```python
from build123d import *

# Parameters (mm, degrees)
F1_DEPTH = 40
F2_T     = -5
F4_D     = 80
F4_DEPTH = 60


with BuildPart() as f1:
    # F0 (on Top) → F1 (new body)
    with BuildSketch(Plane.XY):
        Polygon((-170, 270), (-170, 0), (-170, -270), (170, -270), (170, 270), align=None)
    extrude(amount=F1_DEPTH)

    # F2
    f2_openings = [f1.faces().sort_by_distance(p)[0] for p in [
        (0, 0, 40),
    ]]
    offset(amount=F2_T, openings=f2_openings)

    # F4
    with Locations(Plane.XY.offset(5)):
        with Locations((120, 220)):
            Hole(F4_D / 2, depth=F4_DEPTH)


solid = f1.part
```
Could you check a few things on this model? Use its own coordinates, in mm. A direction names the side the tool comes from. Round coordinates to 2 decimals unless told otherwise and drop trailing zeros. Order: outer loops, then holes, each group sorted by start corner. A loop starts at its lowest first (then second) coordinate and runs counter-clockwise, first axis right, second up. Notation, with made-up numbers: (12, -24.75) -> (25, -24.75) arc R25 ccw to (25, 14.25) -> close; hole circle Ø11 at (79, 59). An arc over 180 degrees is marked (long way). One line per question, with ' | ' between items.
Q1. We'd pull the mould along X, two halves only. Please class faces 1 (the face through (-170, 4, 20)), 2 (the face through (-165, 4, 22)), 3 (the face through (2, 270, 20)): released by +X, released by -X, zero draft, split by the parting line, or undercut.
Computed values:
face 1: released by -X | face 2: undercut | face 3: zero draft
Q2. I'm going to push flat-ended pins straight in: pin 1 (1.5 mm diameter, centred on x = 125, y = 173.5, fed in from -Z); pin 2 (12 mm diameter, centred on x = 74.5, y = 178, fed in from +Z). Where does each tip first touch, or does it pass through?
Computed values:
pin 1: z = 0 | pin 2: z = 5
Q3. If we section it at A-A on x = 120: Write out the boundary of the cut face in (y, z), plus the area to 3 significant figures.
Computed values:
outline: (-270, 0) -> (180, 0) -> (180, 5) -> (-265, 5) -> (-265, 40) -> (-270, 40) -> close; (260, 0) -> (270, 0) -> (270, 40) -> (265, 40) -> (265, 5) -> (260, 5) -> close | area: 2,650 mm²
Q4. If we section it at B-B on z = 24: Write out the boundary of the cut face in (x, y), plus the area to 3 significant figures.
Computed values:
outline: (-170, -270) -> (170, -270) -> (170, 270) -> (-170, 270) -> close; hole (-165, -265) -> (165, -265) -> (165, 265) -> (-165, 265) -> close | area: 8,700 mm²
Q5. If we section it at D-D on y = 129: Write out the boundary of the cut face in (x, z), plus the area to 3 significant figures.
Computed values:
outline: (-170, 0) -> (170, 0) -> (170, 40) -> (165, 40) -> (165, 5) -> (-165, 5) -> (-165, 40) -> (-170, 40) -> close | area: 2,050 mm²
Q6. If we section it at C-C on y = 220: Write out the boundary of the cut face in (x, z).
Computed values:
outline: (-170, 0) -> (80, 0) -> (80, 5) -> (-165, 5) -> (-165, 40) -> (-170, 40) -> close; (160, 0) -> (170, 0) -> (170, 40) -> (165, 40) -> (165, 5) -> (160, 5) -> close
Q7. Which directions (+Z, -Z, +X, -X, +Y, -Y) give clear straight access to the entire face, cutting with the end or side of a thin tool? Please do faces 4 (the face through (-2, -270, 20)), 5 (the face through (-2, -265, 22)).
Computed values:
face 4: +Z, -Z, +X, -X, -Y | face 5: +Z
Q8. If I drill on line 1 (Y direction, x = -29.5, z = 26.5); line 2 (X direction, y = 149.5, z = 38.5); line 3 (Y direction, x = 120, z = 2), over which ranges is the centre line in solid material (lowest first)? Write a range as from..to.
Computed values:
line 1: -270..-265, 265..270 | line 2: -170..-165, 165..170 | line 3: -270..180, 260..270
